Build history of the part. All positions in model axes, mm. Face numbers are marked on the shaded views. A direction names the side the tool comes from. Round coordinates to 2 decimals unless told otherwise and drop trailing zeros. Loops run counter-clockwise (first coordinate to the right, second up) from the corner with the lowest first, then second, coordinate; pieces in that order, holes last. Notation, with made-up numbers: (52.5, -4.75) -> (111.5, -4.75) arc R21 cw to (111.5, 26.25) -> close; hole circle Ø3 at (-28.75, 11). An arc over 180 degrees is marked (long way). Put each result on its own line as item: value. Start each with the question number.
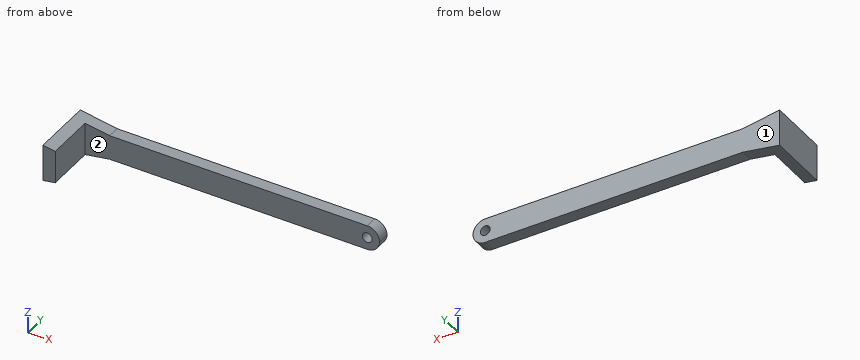
Autodesk Inventor part; units mm, degrees
ref_plane "YZ Plane" through (0, 0, 0) normal (1, 0, 0) x (0, 1, 0)
ref_plane "XZ Plane" through (0, 0, 0) normal (0, 1, 0) x (-1, 0, 0)
ref_plane "XY Plane" through (0, 0, 0) normal (0, 0, 1) x (1, 0, 0)
sketch "Schizzo1" plane through (0, 0, 0) normal (0, 0, 1) x (1, 0, 0)
  line L0 (0, 0) -> (0, 50)
  line L1 (0, 50) -> (250, 50)
  line L2 (250, 50) -> (250, 40)
  line L3 (250, 40) -> (10, 40)
  line L4 (10, 40) -> (10, 0)
  line L5 (10, 0) -> (0, 0)
  dimension "d0" = 10
  dimension "d1" = 10
  dimension "d2" = 50
  dimension "d3" = 250
extrude "Estrusione1" add sketch "Schizzo1" along normal blind 30
sketch "Schizzo2" plane through (0, 50, 0) normal (0, 1, 0) x (1, 0, 0)
  circle A0 centre (240, -15) radius 4
  line L0 (250, -30) -> (0, -30)
  line L1 (250, 0) -> (250, -30)
  line L2 (30, 51) -> (328, 51)
  line L3 (328, 51) -> (328, -5)
  line L4 (328, -5) -> (30, -5)
  line L5 (30, 0) -> (30, 51)
  line L6 (336, -124) -> (30, -124)
  line L7 (30, -124) -> (30, -30)
  line L8 (30, -25) -> (336, -25)
  line L9 (336, -25) -> (336, -124)
  line L10 (250, 0) -> (0, 0)
  line L11 (0, 0) -> (0, -30)
  line L12 (30, -5) -> (0, 0)
  line L13 (30, -25) -> (0, -30)
  line L14 (0, 0) -> (328, 124)
  line L15 (328, 124) -> (336, -220)
  line L16 (336, -220) -> (0, -30)
  point P0 (250, -5)
  point P1 (250, -25)
  dimension "d6" = 8
  dimension "d7" = 15
  dimension "d8" = 10
  dimension "d9" = 5
  dimension "d10" = 5
  dimension "d11" = 30
extrude "Estrusione2" cut sketch "Schizzo2" against normal blind 50 contours A0 | L0 L13 L8 L1 | L4 L12 L10 L1
fillet "Raccordo1" radius 10 2 edges at (250, 45, 5) (250, 45, 25)
properties part number "porta penna"
Item 1: 3-axis set-ups, long thin cutter, end or side, ignore diameter. For the marked faces 1 and 2: which of +Z, -Z, +X, -X, +Y, -Y reach the whole face in a straight line?
Item 2: Drop flat-ended pins along their axis: pin 1 (6 mm diameter, centred on y = 17, z = 21.5, fed in from +X); pin 2 (10 mm diameter, centred on x = 30, y = 36, fed in from -Z); pin 3 (5 mm diameter, centred on x = 106.5, z = 21, fed in from -Y). Give the stop position or say it passes through.
Item 3: Cut at D-D on z = 21.75. Write the cut outline in (x, y), then the cut area to 3 significant figures.
Item 4: Cut at B-B on x = 99.5. Write the cut outline in (y, z), then the cut area to 3 significant figures.
Item 5: Cut at C-C on y = 27.5. Write the cut outline in (x, z), then the cut area to 3 significant figures.
Item 6: Wall check: line 1 (Z direction, x = 240, y = 44); line 2 (X direction, y = 46.75, z = 15); line 3 (X direction, y = 24.5, z = 16.25). Give the ranges that are in metal, low to high. Write a range as from..to.
Ans:
1. face 1: +Z, -Z, +X, -X, +Y
1. face 2: +Z, -Z, +X, -Y
2. pin 1: stops at x = 10
2. pin 2: stops at z = 4.5
2. pin 3: stops at y = 40
3. outline: (0, 0) -> (10, 0) -> (10, 40) -> (247.38, 40) -> (247.38, 50) -> (0, 50) -> close
3. area: 2,870 mm2
4. outline: (40, 5) -> (50, 5) -> (50, 25) -> (40, 25) -> close
4. area: 200 mm2
5. outline: (0, 0) -> (10, 1.67) -> (10, 28.33) -> (0, 30) -> close
5. area: 283 mm2
6. line 1: z = 5..11, 19..25
6. line 2: x = 0..236, 244..250
6. line 3: x = 0..10
